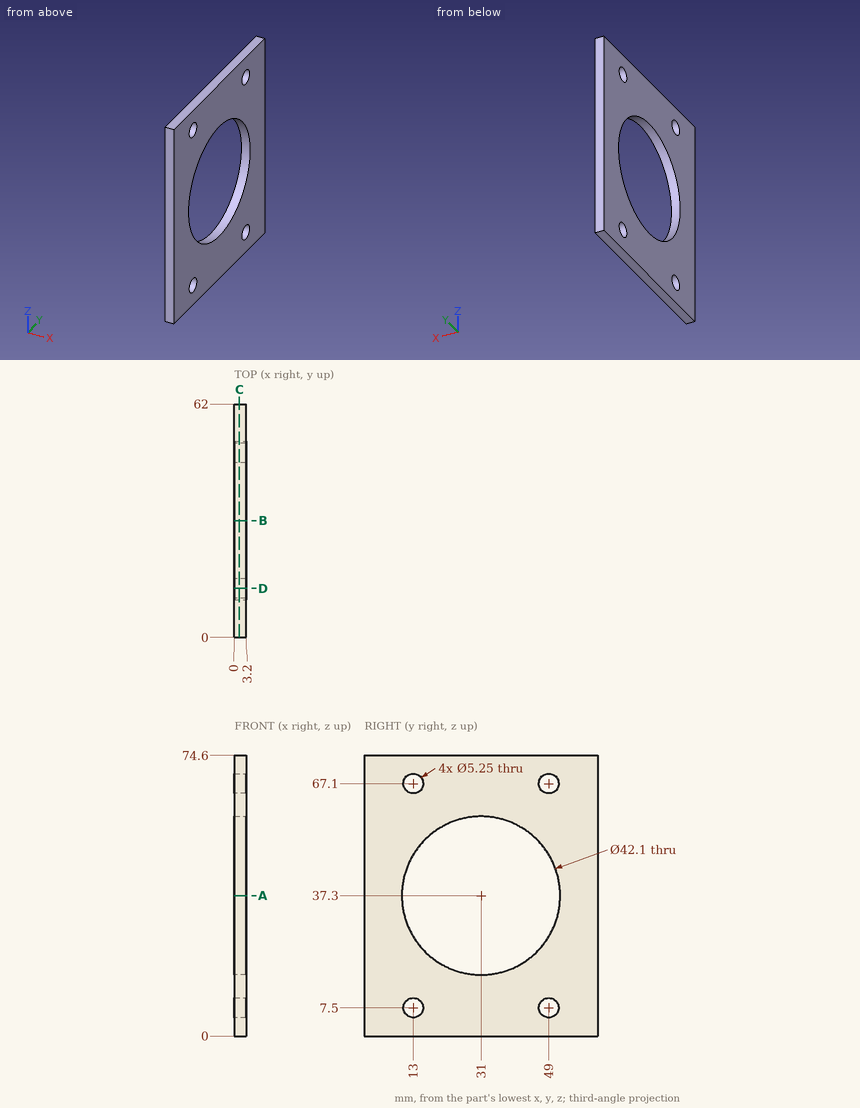
Check sheet for the drawn part. Datum: minimum x, y, z corner. Units: mm. Give positions to 0.01 mm unless a question says otherwise; leave off trailing zeros. Order: outer loops, then holes, each group sorted by start corner. A loop starts at its lowest first (then second) coordinate and runs counter-clockwise, first axis right, second up. Notation, with made-up numbers: (18, 58.25) - (22, 58.25) arc R30 ccw to (22, 82.25) - close; hole circle Ø5 at (61, 33). An arc over 180 degrees is marked (long way). Write item = value, one per line. Start each with the question number.
1) Section check A-A (z = 37.3). Enter the section's corners in (x, y).
2) Section check C-C (x = 1.35). Enter the section's corners in (y, z) (3 decimals), then the cut area to 3 significant figures.
3) Section check D-D (y = 13). Enter the section's corners in (x, z) (3 decimals).
4) Section check B-B (y = 31). Enter the section's corners in (x, z).
5) Scan lines: L1, parallel to Y at x = 2.2, z = 37.3; L2, parallel to Y at x = 1.9, z = 67.1 (3 decimals); L3, parallel to Z at x = 0.9, y = 14. Record each from-to range of solid material in increasing order.
Geometry check:
q1.outline = (0, 0) - (3.2, 0) - (3.2, 9.95) - (0, 9.95) - close; (0, 52.05) - (3.2, 52.05) - (3.2, 62) - (0, 62) - close
q2.outline = (0, 0) - (62, 0) - (62, 74.6) - (0, 74.6) - close; hole circle Ø42.1 at (31, 37.3); hole circle Ø5.25 at (13, 7.5); hole circle Ø5.25 at (13, 67.1); hole circle Ø5.25 at (49, 7.5); hole circle Ø5.25 at (49, 67.1)
q2.area = 3,150 mm2
q3.outline = (0, 0) - (3.2, 0) - (3.2, 4.875) - (0, 4.875) - close; (0, 10.125) - (3.2, 10.125) - (3.2, 26.387) - (0, 26.387) - close; (0, 48.213) - (3.2, 48.213) - (3.2, 64.475) - (0, 64.475) - close; (0, 69.725) - (3.2, 69.725) - (3.2, 74.6) - (0, 74.6) - close
q4.outline = (0, 0) - (3.2, 0) - (3.2, 16.25) - (0, 16.25) - close; (0, 58.35) - (3.2, 58.35) - (3.2, 74.6) - (0, 74.6) - close
q5.L1 = 0 to 9.95, 52.05 to 62
q5.L2 = 0 to 10.375, 15.625 to 46.375, 51.625 to 62
q5.L3 = 0 to 5.07, 9.93 to 24.89, 49.71 to 64.67, 69.53 to 74.6
